Autodesk Inventor part; units mm, degrees
ref_plane "YZ Plane" through (0, 0, 0) normal (1, 0, 0) x (0, 1, 0)
ref_plane "XZ Plane" through (0, 0, 0) normal (0, 1, 0) x (-1, 0, 0)
ref_plane "XY Plane" through (0, 0, 0) normal (0, 0, 1) x (1, 0, 0)
sketch "Skizze1" plane through (0, 0, 0) normal (0, 0, 1) x (1, 0, 0)
  line L0 (12.8939, 32.0057) -> (2.8939, 32.0057)
  line L1 (2.8939, 32.0057) -> (2.8939, 29.0057)
  line L2 (2.8939, 29.0057) -> (12.8939, 29.0057)
  line L3 (12.8939, 29.0057) -> (12.8939, 32.0057)
  line L4 (12.8939, 9.0723) -> (2.8939, 9.0723)
  line L5 (2.8939, 9.0723) -> (2.8939, 6.0723)
  line L6 (2.8939, 6.0723) -> (12.8939, 6.0723)
  line L7 (12.8939, 6.0723) -> (12.8939, 9.0723)
  line L8 (2.8939, 15.6723) -> (12.8939, 15.6723)
  line L9 (12.8939, 15.6723) -> (12.8939, 22.4057)
  line L10 (12.8939, 22.4057) -> (2.8939, 22.4057)
  line L11 (2.8939, 22.4057) -> (2.8939, 15.6723)
  line L12 (2.8939, 9.0723) -> (2.8939, 15.6723) construction
  line L13 (2.8939, 22.4057) -> (2.8939, 29.0057) construction
  point P0 (0, 0)
  point P1 (7.8939, 9.0723)
  dimension "d0" = 10
  dimension "d1" = 3
  dimension "d2" = 3
  dimension "d35" = 25.9333
  dimension "d38" = 6.6
  dimension "d39" = 6.7333
extrude "Extrusion1" add sketch "Skizze1" along normal blind 20
fillet "Rundung1" radius 3 6 edges at (12.8939, 7.5723, 20) (12.8939, 30.5057, 20) (2.8939, 30.5057, 20) (2.8939, 7.5723, 20) (12.8939, 19.039, 20) (2.8939, 19.039, 20)
sketch "Skizze2" plane through (2.8939, 6.0723, 0) normal (0, -1, 0) x (1, 0, 0)
  circle A0 centre (5, 15) radius 5 construction
  line L0 (10, 0) -> (10, 17) construction
  line L1 (0, 0) -> (0, 17) construction
  line L2 (3, 20) -> (7, 20) construction
  point P0 (-2.8939, 0)
hole "Bohrung1" at (7.8939, 6.0723, 15) direction (0, 1, 0) diameter 3.242 end through all countersink diameter 9 countersink angle 90
sketch "Skizze3" plane through (2.8939, 29.0057, 0) normal (0, -1, 0) x (1, 0, 0)
  line L0 (0, 0) -> (10, 0)
  line L1 (10, 0) -> (10, 2)
  line L2 (10, 0) -> (10, 17)
  line L3 (10, 2) -> (0, 2)
  line L4 (0, 0) -> (0, 17)
  point P0 (-2.8939, 0)
  dimension "d15" = 2
extrude "Extrusion2" add sketch "Skizze3" along normal through all
sketch "Skizze4" plane through (2.8939, 29.0057, 2) normal (0, 0, 1) x (1, 0, 0)
  line L0 (5, -16.6333) -> (10, -16.6333) construction
  line L1 (10, -16.6333) -> (10, 0) construction
  line L2 (10, -16.6333) -> (10, -19.9333) construction
  line L3 (5, -3.3) -> (0, -3.3) construction
  line L4 (0, 0) -> (0, -3.3) construction
  line L5 (5, -16.6333) -> (0, -16.6333) construction
  line L6 (0, 0) -> (0, -19.9333) construction
  point P0 (-2.8939, -29.0057)
  dimension "d34" = 13.3333
hole "Bohrung2" at (7.8939, 25.7057, 2) at (7.8939, 12.3723, 2) direction (0, 0, -1) diameter 2 end through all countersink diameter 5 countersink angle 90
sketch "Skizze5" plane through (2.8939, 6.0723, 0) normal (0, -1, 0) x (1, 0, 0)
  circle A0 centre (5, 15) radius 4.5
  point P0 (-2.8939, 0)
hole "Bohrung3" at (7.8939, 6.0723, 15) direction (0, 1, 0) diameter 4 depth 22.9333
properties part number "HalterUmlenkrolleDPL" material "PC/ABS-Kunststoff, 3DDruck, PLA"
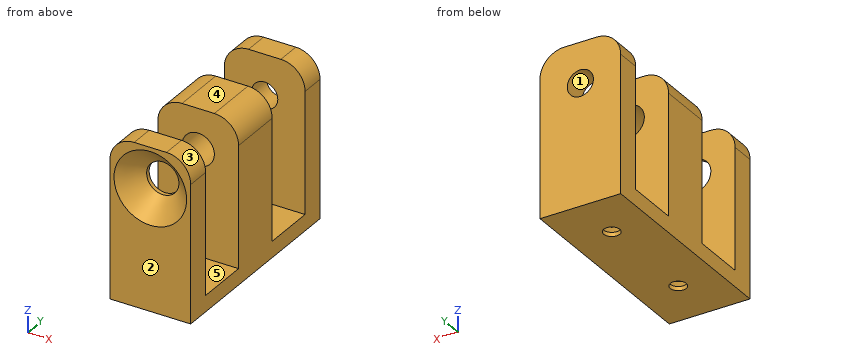
Geometry: final body of the model. Coordinates: model frame, mm. Face numbers are marked on the shaded views. A direction names the side the tool comes from. Coordinates: 2 decimals unless noted, no trailing zeros. Order: outer loops, then holes, each group sorted by start corner. A loop starts at its lowest first (then second) coordinate and runs counter-clockwise, first axis right, second up. Notation, with made-up numbers: M 46.5,-15 L 51.5,-15 A33 cw 51.5,24 Z; hole C 30.25,29.25 d3. An arc over 180 degrees is marked long. Answer in a Markdown table with one row per item. Add a question column.
Q1. Section query C-C on y = 16.5. Return the cut outline in (x, z).
Q2. Reachability of the marked faces 4 and 5 from +Z, -Z, +X, -X, +Y, -Y: full face, straight path, thin tool, end or side. Return the list, or none.
Q3. Contact query for flat-ended pins moving along their axis: P1, Ø2.5, axis at x = 7.89, y = 12.37, coming from the -Z side; P2, Ø2, axis at x = 7.5, y = 24.5, coming from the +Z side; P3, Ø2.5, axis at x = 7.89, y = 25.71, coming from the +Z side; P4, Ø2, axis at x = 9, y = 11, coming from the +Z side. Output: stop coordinate, or through.
Q4. Mould query, pull axis X, two halves, no side actions, for the marked faces 1, 2 and 3. Classes: released by +X, released by -X, zero draft, split by the parting line, or undercut.
Q5. Line query: L1, parallel to Y at x = 7, z = 3.75; L2, parallel to X at y = 20.5, z = 15; L3, parallel to Y at x = 11.75, z = 16.25. Output: solid intervals per line, ascending.
Q6. Section query A-A on z = 4.75. Return the cut outline in (x, y).
Q7. Section query D-D on y = 9.5. Return the cut outline in (x, z).
Q8. Section query B-B on z = 15. Return the cut outline in (x, y).
Completed:
| question | item | result |
|---|---|---|
| 1 | outline | M 2.89,0 L 12.89,0 L 12.89,17 A3 ccw 9.89,20 L 5.89,20 A3 ccw 2.89,17 Z; hole C 7.89,15 d4 |
| 2 | face 4 | +Z, +X, -X, +Y, -Y |
| 2 | face 5 | +Z, +X, -X |
| 3 | P1 | stops at z = 0 |
| 3 | P2 | stops at z = 1.77 |
| 3 | P3 | stops at z = 0.76 |
| 3 | P4 | stops at z = 2 |
| 4 | face 1 | undercut |
| 4 | face 2 | zero draft |
| 4 | face 3 | released by +X |
| 5 | L1 | y = 6.07 to 9.07, 15.67 to 22.41, 29.01 to 32.01 |
| 5 | L2 | x = 2.89 to 5.89, 9.89 to 12.89 |
| 5 | L3 | y = 6.52 to 9.07, 15.67 to 22.41, 29.01 to 32.01 |
| 6 | outline | M 2.89,6.07 L 12.89,6.07 L 12.89,9.07 L 2.89,9.07 Z; M 2.89,15.67 L 12.89,15.67 L 12.89,22.41 L 2.89,22.41 Z; M 2.89,29.01 L 12.89,29.01 L 12.89,32.01 L 2.89,32.01 Z |
| 7 | outline | M 2.89,0 L 12.89,0 L 12.89,2 L 2.89,2 Z |
| 8 | outline | M 2.89,6.07 L 3.39,6.07 L 5.89,8.57 L 5.89,9.07 L 2.89,9.07 Z; M 2.89,15.67 L 5.89,15.67 L 5.89,22.41 L 2.89,22.41 Z; M 2.89,29.01 L 6.27,29.01 L 6.27,32.01 L 2.89,32.01 Z; M 9.51,29.01 L 12.89,29.01 L 12.89,32.01 L 9.51,32.01 Z; M 9.89,8.57 L 12.39,6.07 L 12.89,6.07 L 12.89,9.07 L 9.89,9.07 Z; M 9.89,15.67 L 12.89,15.67 L 12.89,22.41 L 9.89,22.41 Z |
